Can you work these out from the model? Positions are in its coordinate system, mm. A direction names the side the tool comes from. Coordinates: 2 decimals unless noted, no trailing zeros. Loops run counter-clockwise (first coordinate to the right, second up) from the corner with the lowest first, then second, coordinate; pieces in that order, holes last. Notation, with made-up numbers: M -36,56.25 L 1,56.25 A29 cw 1,79.25 Z; hole C 43.25,38 d9. An arc over 180 degrees is marked long. Answer as a JSON object with one key per item and string values. Group by question number.
Item 1: We'd pull the mould along X, two halves only. Please class faces 5 (the flat face through (-95, 3, -21)), 6 (the cylindrical face through (-83.031, 12.146, -28.552)), 7 (the flat face through (63, 9, -32)): +X half, -X half, draft (parallel to the pull), parting line (faces both ways), or undercut.
Item 2: Suppose I cut it at B-B (x = -39.5). Write out the boundary of the cut face in (y, z), then the cut area to 3 significant figures.
Item 3: If I drill on line 1 (X direction, y = 11.5, z = -27); line 2 (Z direction, x = 13.5, y = 1.25); line 3 (X direction, y = 18, z = -27.5), over which ranges is the centre line in solid material (lowest first)?
Item 4: Suppose I cut it at A-A (y = 6). Write out the boundary of the cut face in (x, z).
Item 5: I'm going to push flat-ended pins straight in: pin 1 Ø8 at (x, y) = (-60, 10.5) entering from +Z; pin 2 Ø2 at (x, y) = (-27, 1.5) entering from -Z; pin 3 Ø5 at (x, y) = (65, 11.5) entering from -Z; pin 4 Ø3.5 at (x, y) = (-86.5, 11) entering from +Z. Where does each tip first touch, or does it pass through?
Item 6: Suppose I cut it at C-C (x = -65). Write out the boundary of the cut face in (y, z).
Item 7: Which directions (+Z, -Z, +X, -X, +Y, -Y) give clear straight access to the entire face, cutting with the end or side of a thin tool? Please do faces 1 (the flat face through (65, 15.15, -24)), 2 (the flat face through (-75, 11, -22)), 3 (the flat face through (1, 2, -10)), 4 (the flat face through (1, 2, 5)).
```python
from build123d import *

# Parameters (mm, degrees)
SKIZZE1_W                       = 55
SKIZZE1_H                       = 5
AUFSATZ_LINEAR_AUSTRAGEN1_DEPTH = 4
AUFSATZ_LINEAR_AUSTRAGEN2_DEPTH = 15
SCHNITT_LINEAR_AUSTRAGEN1_DEPTH = 3.2
SCHNITT_LINEAR_AUSTRAGEN2_DEPTH = 15


with BuildPart() as part:
    # Skizze1 → Aufsatz-Linear austragen1 (new body)
    with BuildSketch(Plane(origin=(0, 0, 0), x_dir=(1, 0, 0), z_dir=(0, 1, 0))):
        with BuildLine():
            Line((-55, -5), (-55, 0))
            Line((-55, 0), (-72.85, 0))
            ThreePointArc((-72.85, 0), (-76.52027958, -1.52027958), (-75, 2.15))
            Line((-75, 2.15), (-75, 27.9))
            ThreePointArc((-75, 27.9), (-77.899137803, 29.100862197), (-79.1, 32))
            Line((-79.1, 32), (-95, 32))
            Line((-95, 32), (-95, -10))
            Line((-95, -10), (-55, -10))
            Line((-55, -10), (-55, -5))
        make_face()
        with BuildLine():
            Line((-72.85, 0), (-55, 0))
            Line((-55, 0), (-55, 5))
            Line((-55, 5), (-55, 10))
            Line((-55, 10), (-55, 32))
            Line((-55, 32), (-70.9, 32))
            ThreePointArc((-70.9, 32), (-72.100862197, 29.100862197), (-75, 27.9))
            Line((-75, 27.9), (-75, 2.15))
            ThreePointArc((-75, 2.15), (-73.47972042, 1.52027958), (-72.85, 0))
        make_face()
        with Locations((-27.5, 7.5)):
            Rectangle(SKIZZE1_W, SKIZZE1_H)
        with Locations((27.5, 7.5)):
            Rectangle(SKIZZE1_W, SKIZZE1_H)
        with BuildLine():
            Line((55, 5), (55, 0))
            Line((55, 0), (72.85, 0))
            ThreePointArc((72.85, 0), (73.47972042, 1.52027958), (75, 2.15))
            Line((75, 2.15), (75, 27.9))
            ThreePointArc((75, 27.9), (72.100862197, 29.100862197), (70.9, 32))
            Line((70.9, 32), (55, 32))
            Line((55, 32), (55, 10))
            Line((55, 10), (55, 5))
        make_face()
        with BuildLine():
            Line((72.85, 0), (55, 0))
            Line((55, 0), (55, -5))
            Line((55, -5), (55, -10))
            Line((55, -10), (95, -10))
            Line((95, -10), (95, 32))
            Line((95, 32), (79.1, 32))
            ThreePointArc((79.1, 32), (77.899137803, 29.100862197), (75, 27.9))
            Line((75, 27.9), (75, 2.15))
            ThreePointArc((75, 2.15), (76.52027958, 1.52027958), (77.15, 0))
            ThreePointArc((77.15, 0), (75, -2.15), (72.85, 0))
        make_face()
        with Locations((27.5, -7.5)):
            Rectangle(SKIZZE1_W, SKIZZE1_H)
        with Locations((-27.5, -7.5)):
            Rectangle(SKIZZE1_W, SKIZZE1_H)
    extrude(amount=AUFSATZ_LINEAR_AUSTRAGEN1_DEPTH)

    # Skizze2 → Aufsatz-Linear austragen2 (add)
    with BuildSketch(Plane(origin=(0, 4, 0), x_dir=(1, 0, 0), z_dir=(0, 1, 0))):
        with BuildLine():
            Line((-95, 32), (-95, 22))
            Line((-95, 22), (-55, 22))
            Line((-55, 22), (-55, 32))
            Line((-55, 32), (-70.9, 32))
            ThreePointArc((-70.9, 32), (-75, 27.9), (-79.1, 32))
            Line((-79.1, 32), (-95, 32))
        make_face()
        with BuildLine():
            Line((55, 32), (55, 22))
            Line((55, 22), (95, 22))
            Line((95, 22), (95, 32))
            Line((95, 32), (79.1, 32))
            ThreePointArc((79.1, 32), (75, 27.9), (70.9, 32))
            Line((70.9, 32), (55, 32))
        make_face()
    extrude(amount=AUFSATZ_LINEAR_AUSTRAGEN2_DEPTH)

    # Skizze3 → Schnitt-Linear austragen1 (cut)
    with BuildSketch(Plane.XY.offset(-22)):
        Polygon((-87.107328483, 15.15), (-89.214656965, 11.5), (-85, 11.5), (-80.785343035, 11.5), (-82.892671517, 15.15), align=None)
        Polygon((-85, 11.5), (-89.214656965, 11.5), (-87.107328483, 7.85), (-82.892671517, 7.85), (-80.785343035, 11.5), align=None)
        Polygon((-67.107328483, 15.15), (-69.214656965, 11.5), (-65, 11.5), (-60.785343035, 11.5), (-62.892671517, 15.15), align=None)
        Polygon((-65, 11.5), (-69.214656965, 11.5), (-67.107328483, 7.85), (-62.892671517, 7.85), (-60.785343035, 11.5), align=None)
        Polygon((85, 11.5), (89.214656965, 11.5), (87.107328483, 15.15), (82.892671517, 15.15), (80.785343035, 11.5), align=None)
        Polygon((87.107328483, 7.85), (89.214656965, 11.5), (85, 11.5), (80.785343035, 11.5), (82.892671517, 7.85), align=None)
        Polygon((65, 11.5), (69.214656965, 11.5), (67.107328483, 15.15), (62.892671517, 15.15), (60.785343035, 11.5), align=None)
        Polygon((67.107328483, 7.85), (69.214656965, 11.5), (65, 11.5), (60.785343035, 11.5), (62.892671517, 7.85), align=None)
    extrude(amount=-SCHNITT_LINEAR_AUSTRAGEN1_DEPTH, mode=Mode.SUBTRACT)

    # Skizze4 → Schnitt-Linear austragen2 (cut)
    with BuildSketch(Plane.XY.offset(-22)):
        with BuildLine():
            ThreePointArc((-87.231768347, 11.5), (-85.081768347, 9.35), (-82.931768347, 11.5))
            Line((-82.931768347, 11.5), (-85.081768347, 11.5))
            Line((-85.081768347, 11.5), (-87.231768347, 11.5))
        make_face()
        with BuildLine():
            Line((-85.081768347, 11.5), (-82.931768347, 11.5))
            ThreePointArc((-82.931768347, 11.5), (-85.081768347, 13.65), (-87.231768347, 11.5))
            Line((-87.231768347, 11.5), (-85.081768347, 11.5))
        make_face()
        with BuildLine():
            ThreePointArc((-67.15, 11.5), (-65, 9.35), (-62.85, 11.5))
            Line((-62.85, 11.5), (-65, 11.5))
            Line((-65, 11.5), (-67.15, 11.5))
        make_face()
        with BuildLine():
            Line((-65, 11.5), (-62.85, 11.5))
            ThreePointArc((-62.85, 11.5), (-65, 13.65), (-67.15, 11.5))
            Line((-67.15, 11.5), (-65, 11.5))
        make_face()
        with BuildLine():
            ThreePointArc((62.85, 11.5), (65, 9.35), (67.15, 11.5))
            Line((67.15, 11.5), (65, 11.5))
            Line((65, 11.5), (62.85, 11.5))
        make_face()
        with BuildLine():
            Line((65, 11.5), (67.15, 11.5))
            ThreePointArc((67.15, 11.5), (65, 13.65), (62.85, 11.5))
            Line((62.85, 11.5), (65, 11.5))
        make_face()
        with BuildLine():
            ThreePointArc((82.85, 11.5), (85, 9.35), (87.15, 11.5))
            Line((87.15, 11.5), (85, 11.5))
            Line((85, 11.5), (82.85, 11.5))
        make_face()
        with BuildLine():
            Line((85, 11.5), (87.15, 11.5))
            ThreePointArc((87.15, 11.5), (85, 13.65), (82.85, 11.5))
            Line((82.85, 11.5), (85, 11.5))
        make_face()
    extrude(amount=-SCHNITT_LINEAR_AUSTRAGEN2_DEPTH, mode=Mode.SUBTRACT)


solid = part.part
```
From the geometry:
{
 "1": {"face 5": "-X half", "face 6": "undercut", "face 7": "draft"},
 "2": {"outline": "M 0,-10 L 4,-10 L 4,-5 L 0,-5 Z; M 0,5 L 4,5 L 4,10 L 0,10 Z", "area": "40.0 mm2"},
 "3": {"line 1": "-95 to -87.23, -82.93 to -67.15, -62.85 to -55, 55 to 62.85, 67.15 to 82.85, 87.15 to 95", "line 2": "-10 to -5, 5 to 10", "line 3": "-95 to -55, 55 to 95"},
 "4": {"outline": "M -95,-32 L -79.1,-32 A4.1 cw -70.9,-32 L -55,-32 L -55,-22 L -95,-22 Z; M 55,-32 L 70.9,-32 A4.1 cw 79.1,-32 L 95,-32 L 95,-22 L 55,-22 Z"},
 "5": {"pin 1": "z = -22", "pin 2": "z = -10", "pin 3": "z = -32", "pin 4": "z = -25.2"},
 "6": {"outline": "M 0,-32 L 9.35,-32 L 9.35,-25.2 L 7.85,-25.2 L 7.85,-22 L 4,-22 L 4,10 L 0,10 Z; M 13.65,-32 L 19,-32 L 19,-22 L 15.15,-22 L 15.15,-25.2 L 13.65,-25.2 Z"},
 "7": {"face 1": "+Z", "face 2": "+Z, +X, -X, +Y", "face 3": "-Z, +Y, -Y", "face 4": "+Y, -Y"}
}
